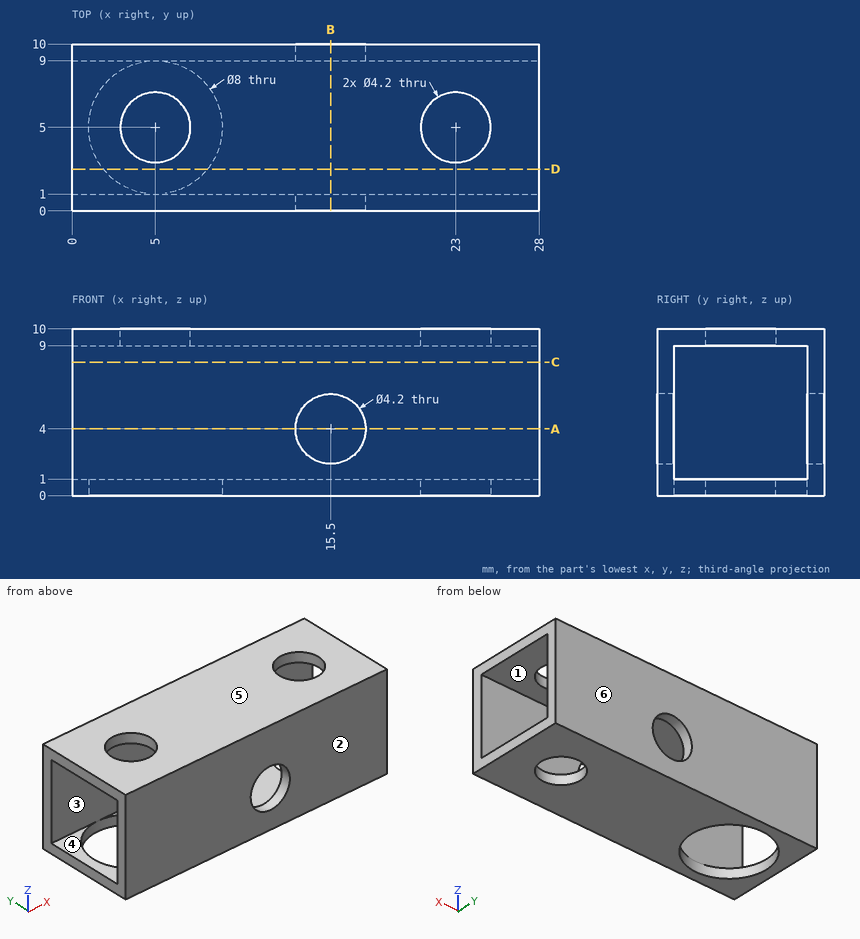
Geometry check sheet. Reference: drawing and pictorial views, mm from the part's lowest x, y, z. A direction names the side the tool comes from. Coordinates: 2 decimals unless noted, no trailing zeros. Order: outer loops, then holes, each group sorted by start corner. A loop starts at its lowest first (then second) coordinate and runs counter-clockwise, first axis right, second up. Notation, with made-up numbers: M 74,43.25 L 132,43.25 A17 ccw 132,64.25 Z; hole C 79,76.25 d1. An arc over 180 degrees is marked long. Return JSON: item names as keys, results as strings.
1) Access from +Z, -Z, +X, -X, +Y, -Y to the whole of each face (thin tool, end or side, straight path). Record for the marked faces 1 and 2.
Answer list:
{"face 1": "+X, -X", "face 2": "+Z, -Z, +X, -X, -Y"}
2) Cross-section at B-B, the plane x = 15.5. Record the boundary of the cut face in (y, z), and give its area (3 significant figures).
Answer list:
{"outline": "M 0,0 L 10,0 L 10,1.9 L 9,1.9 L 9,1 L 1,1 L 1,1.9 L 0,1.9 Z; M 0,6.1 L 1,6.1 L 1,9 L 9,9 L 9,6.1 L 10,6.1 L 10,10 L 0,10 Z", "area": "27.6 mm2"}
3) Cross-section at A-A, the plane z = 4. Record the boundary of the cut face in (x, y).
Answer list:
{"outline": "M 0,0 L 13.4,0 L 13.4,1 L 0,1 Z; M 0,9 L 13.4,9 L 13.4,10 L 0,10 Z; M 17.6,0 L 28,0 L 28,1 L 17.6,1 Z; M 17.6,9 L 28,9 L 28,10 L 17.6,10 Z"}
4) Thickness scan on L1, parallel to Y at x = 23, z = 0.4; L2, parallel to Y at x = 23.5, z = 2.75. Record the ranges inside material, lowest first. Write a range as [from, to].
Answer list:
{"L1": "[0, 2.9], [7.1, 10]", "L2": "[0, 1], [9, 10]"}
5) Cross-section at C-C, the plane z = 8. Record the boundary of the cut face in (x, y).
Answer list:
{"outline": "M 0,0 L 28,0 L 28,1 L 0,1 Z; M 0,9 L 28,9 L 28,10 L 0,10 Z"}
6) Cross-section at D-D, the plane y = 2.5. Record the boundary of the cut face in (x, z).
Answer list:
{"outline": "M 0,0 L 1.88,0 L 1.88,1 L 0,1 Z; M 0,9 L 28,9 L 28,10 L 0,10 Z; M 8.12,0 L 28,0 L 28,1 L 8.12,1 Z"}
7) Gauge pin test, flat end, axial feed: pin 1 (4 mm diameter, centred on x = 23, y = 5, fed in from -Z). Record the tip position at first contact, or that the pin passes through.
Answer list:
{"pin 1": "through"}
8) Release check for a two-part mould opening along Z. For the marked faces 3, 4, 5 and 6 record: +Z half, -Z half, draft (parallel to the pull), parting line (faces both ways), or undercut.
Answer list:
{"face 3": "undercut", "face 4": "undercut", "face 5": "+Z half", "face 6": "draft"}
